from build123d import *

# Parameters (mm, degrees)
F0_W     = 127
F0_H     = 127
F1_DEPTH = 127
F2_R     = 38.1
F3_DEPTH = 127.001
F4_R     = 38.1
F5_DEPTH = 127.001


with BuildPart() as f1:
    # F0 (on Front) → F1 (new body)
    with BuildSketch(Plane.XZ):
        with Locations((-0.983404, -0.074951)):
            Rectangle(F0_W, F0_H)
    extrude(amount=F1_DEPTH)

    # F2 (on face) → F3 (cut, through all)
    with BuildSketch(Plane.XZ.offset(127)):
        Circle(F2_R)
    extrude(amount=-F3_DEPTH, mode=Mode.SUBTRACT)

    # F4 (on face) → F5 (cut, through all)
    with BuildSketch(Plane.YZ.offset(62.516596)):
        with Locations((-63.5, 0)):
            Circle(F4_R)
    extrude(amount=-F5_DEPTH, mode=Mode.SUBTRACT)


solid = f1.part
Verification items for the finished model (mm, model axes). Give positions to 0.01 mm unless a question says otherwise; leave off trailing zeros. Write each loop counter-clockwise with the first axis right and the second up, starting at its lowest first coordinate (ties: lowest second). Pieces come first, ordered by that corner, then holes.
(1) Material ranges on line 1 (Z direction, x = -13, y = -63.5); line 2 (Y direction, x = 34, z = -29); line 3 (Y direction, x = -45, z = -10), recorded low to high.
(2) Mould release check, pull along Z, two halves, no side actions. Record for faces 1 (the face through (-8.259, -102.75, -37.194)), 2 (the face through (-2, -63, -63.575)), 3 (the face through (-30, -127, 29)), 4 (the face through (38.642, -71.759, -37.194)): +Z half, -Z half, draft (parallel to the pull), parting line (faces both ways), or undercut.
(3) Cross-section at B-B (y = -69). Enter the section's corners in (x, z), plus the area to 3 significant figures.
(4) Cross-section at D-D (z = -27.5). Enter the section's corners in (x, y).
(5) Cross-section at A-A (z = 0). Enter the section's corners in (x, y).
(6) Cross-section at C-C (x = 4). Enter the section's corners in (y, z), plus the area to 3 significant figures.
Worked out:
1. line 1: z = -63.57 to -38.1, 38.1 to 63.43
1. line 2: y = -127 to -88.21, -38.79 to 0
1. line 3: y = -127 to -100.26, -26.74 to 0
2. face 1: undercut
2. face 2: -Z half
2. face 3: draft
2. face 4: undercut
3. outline: (-64.48, -63.57) - (62.52, -63.57) - (62.52, -37.7) - (5.5, -37.7) arc R38.1 cw to (-5.5, -37.7) - (-64.48, -37.7) - close; (-64.48, 37.7) - (-5.5, 37.7) arc R38.1 cw to (5.5, 37.7) - (62.52, 37.7) - (62.52, 63.43) - (-64.48, 63.43) - close
3. area: 6,550 mm2
4. outline: (-64.48, -127) - (-26.37, -127) - (-26.37, -89.87) - (-64.48, -89.87) - close; (-64.48, -37.13) - (-26.37, -37.13) - (-26.37, 0) - (-64.48, 0) - close; (26.37, -127) - (62.52, -127) - (62.52, -89.87) - (26.37, -89.87) - close; (26.37, -37.13) - (62.52, -37.13) - (62.52, 0) - (26.37, 0) - close
5. outline: (-64.48, -127) - (-38.1, -127) - (-38.1, -101.6) - (-64.48, -101.6) - close; (-64.48, -25.4) - (-38.1, -25.4) - (-38.1, 0) - (-64.48, 0) - close; (38.1, -127) - (62.52, -127) - (62.52, -101.6) - (38.1, -101.6) - close; (38.1, -25.4) - (62.52, -25.4) - (62.52, 0) - (38.1, 0) - close
6. outline: (-127, -63.57) - (0, -63.57) - (0, -37.89) - (-59.5, -37.89) arc R38.1 cw to (-67.5, -37.89) - (-127, -37.89) - close; (-127, 37.89) - (-67.5, 37.89) arc R38.1 cw to (-59.5, 37.89) - (0, 37.89) - (0, 63.43) - (-127, 63.43) - close
6. area: 6,500 mm2
